Source: CAD feature listing. Evaluate the final solid. Frame: model axes, mm. A direction names the side the tool comes from. Give positions to 0.01 mm unless a question says otherwise; leave off trailing zeros. Order: outer loops, then holes, each group sorted by start corner. A loop starts at its lowest first (then second) coordinate and runs counter-clockwise, first axis right, second up. Notation, with made-up numbers: (16.25, -18) - (73.25, -18) arc R30 ccw to (73.25, 18) - close; hole circle Ø7 at (-32, 21). An arc over 180 degrees is marked (long way). Write each question's results on one line, items separated by ' | '. Start each with the question number.
Item 1: Line query: line 1 along Z through (x, y) = (-95.5, 4); line 2 along Z through (x, y) = (-545, 9.5); line 3 along X through (y, z) = (5.5, -281.5). Output: solid intervals per line, ascending.
Item 2: Section D-D on y = 7.75. Output: boundary loops of the cut face in (x, z).
Item 3: Contact query for flat-ended pins moving along their axis: pin 1 Ø7.5 at (x, y) = (-285.5, 11) entering from +Z; pin 2 Ø1 at (x, y) = (-388.5, 12.5) entering from +Z. Output: stop coordinate, or through.
Item 4: Section C-C on x = -481.5. Output: boundary loops of the cut face in (y, z).
Item 5: Section A-A on x = -389.5. Output: boundary loops of the cut face in (y, z), and give its area (3 significant figures).
Item 6: Set-up query: faces 1 (the cylindrical face through (-172.518, 7.465, -167.871)), 2 (the flat face through (-540, 7, -25)), 3 (the flat face through (-322, 8, -475)). Return all of +Z, -Z, +X, -X, +Y, -Y with unobstructed straight access to the full face (end or side cutting, diameter ignored); none if empty.
Item 7: Mould query, pull axis X, two halves, no side actions, for faces 4 (the flat face through (-167, 0, -170)), 5 (the flat face through (-36.438, 8, -331)), 6 (the flat face through (-609, 7, -257)). Classes: released by +X, released by -X, zero draft, split by the parting line, or undercut.
Item 8: Section B-B on z = -294. Output: boundary loops of the cut face in (x, y), and give its area (3 significant figures).
Autodesk Fusion 360 part; units mm, degrees
sketch "Sketch1" plane through (0, 0, 0) normal (0, 1, 0) x (1, 0, 0)
  line L0 (-25, 25) -> (-25, 482)
  line L1 (-25, 482) -> (-609, 482)
  line L2 (-609, 482) -> (-609, 25)
  line L3 (-609, 25) -> (-469, 25)
  line L4 (-444, 175) -> (-190, 175)
  line L5 (-469, 25) -> (-469, 150)
  arc A0 (-444, 175) -> (-469, 150) centre (-444, 150) ccw
  line L6 (-165, 25) -> (-25, 25)
  line L7 (-165, 150) -> (-165, 25)
  arc A1 (-165, 150) -> (-190, 175) centre (-190, 150) ccw
  point P0 (-469, 175)
  point P1 (-165, 175)
  dimension "d1" = 457
  dimension "d2" = 584
  dimension "d3" = 457
  dimension "d5" = 304
  dimension "d7" = 25
  dimension "d8" = 25
extrude "Extrude1" add sketch "Sketch1" along normal blind 15
sketch "Sketch2" plane through (0, 15, 0) normal (0, 1, 0) x (-1, 0, 0)
  line L0 (165, -25) -> (25, -25)
  line L1 (25, -25) -> (25, -482)
  line L2 (25, -482) -> (609, -482)
  line L3 (609, -482) -> (609, -25)
  line L4 (609, -25) -> (469, -25)
  line L5 (469, -25) -> (469, -150)
  arc A0 (444, -175) -> (469, -150) centre (444, -150) ccw
  line L6 (444, -175) -> (190, -175)
  arc A1 (165, -150) -> (190, -175) centre (190, -150) ccw
  line L7 (165, -150) -> (165, -25)
  line L8 (600, -475) -> (36.4384, -475)
  line L9 (36.4384, -475) -> (36.4384, -182.5461)
  line L10 (36.4384, -182.5461) -> (600, -182.5461)
  line L11 (600, -182.5461) -> (600, -475)
  dimension "d11" = 563.5616
extrude "Extrude2" cut sketch "Sketch2" against normal blind 10 contours L8 L9 L10 L11
shell "Shell1" thickness 5 removed faces 1 at (-412.1461, 5, -377.5154)
extrude "Extrude3" cut 1 faces at (-412.1461, 5, -377.5154) along direction (0, -1, 0) blind 5
sketch "Sketch3" plane through (0, 15, 0) normal (0, 1, 0) x (-1, 0, 0)
  line L0 (36.4384, -475) -> (36.4384, -182.5461)
  line L1 (36.4384, -182.5461) -> (600, -182.5461)
  line L2 (600, -182.5461) -> (600, -475)
  line L3 (600, -475) -> (36.4384, -475)
  line L4 (165, -25) -> (25, -25)
  line L5 (25, -25) -> (25, -482)
  line L6 (25, -482) -> (609, -482)
  line L7 (609, -482) -> (609, -25)
  line L8 (609, -25) -> (469, -25)
  line L9 (469, -25) -> (469, -150)
  arc A0 (444, -175) -> (469, -150) centre (444, -150) ccw
  line L10 (444, -175) -> (190, -175)
  arc A1 (165, -150) -> (190, -175) centre (190, -150) ccw
  line L11 (165, -150) -> (165, -25)
  circle A2 centre (544.2965, -92.6642) radius 50
  curve A3
  dimension "d17" = 100
  dimension "d18" = 100
extrude "Extrude4" cut sketch "Sketch3" against normal blind 20 contours A2
sketch "Sketch4" plane through (0, 15, 0) normal (0, 1, 0) x (-1, 0, 0)
  circle A0 centre (544.2965, -92.6642) radius 50
  line L0 (36.4384, -475) -> (36.4384, -182.5461)
  line L1 (36.4384, -182.5461) -> (600, -182.5461)
  line L2 (600, -182.5461) -> (600, -475)
  line L3 (600, -475) -> (36.4384, -475)
  line L4 (165, -25) -> (25, -25)
  line L5 (25, -25) -> (25, -482)
  line L6 (25, -482) -> (609, -482)
  line L7 (609, -482) -> (609, -25)
  line L8 (609, -25) -> (469, -25)
  line L9 (469, -25) -> (469, -150)
  arc A1 (444, -175) -> (469, -150) centre (444, -150) ccw
  line L10 (444, -175) -> (190, -175)
  arc A2 (165, -150) -> (190, -175) centre (190, -150) ccw
  line L11 (165, -150) -> (165, -25)
  circle A3 centre (92.6724, -96.5653) radius 50
  dimension "d23" = 100
extrude "Extrude5" cut sketch "Sketch4" against normal blind 20 contours A3
fillet "Fillet1" radius 5 1 edges at (-46.056, 0, -114.6461)
fillet "Fillet2" radius 5 1 edges at (-46.056, 15, -78.4846)
fillet "Fillet3" radius 5 1 edges at (-497.6801, 0, -110.745)
fillet "Fillet4" radius 5 1 edges at (-497.6801, 15, -74.5834)
fillet "Fillet5" radius 5 5 edges at (-469, 15, -87.5) (-461.6777, 15, -167.6777) (-317, 15, -175) (-172.3223, 15, -167.6777) (-165, 15, -87.5)
fillet "Fillet6" radius 5 5 edges at (-469, 0, -87.5) (-461.6777, 0, -167.6777) (-317, 0, -175) (-172.3223, 0, -167.6777) (-165, 0, -87.5)
Evaluation:
1) line 1: z = -482 to -475, -182.55 to -146.59, -46.54 to -25 | line 2: z = -482 to -475, -182.55 to -142.66, -42.67 to -25 | line 3: x = -609 to -600, -36.44 to -25
2) outline: (-609, -482) - (-25, -482) - (-25, -25) - (-165, -25) - (-165, -150) arc R25 cw to (-190, -175) - (-444, -175) arc R25 cw to (-469, -150) - (-469, -25) - (-609, -25) - close; hole (-600, -475) - (-36.44, -475) - (-36.44, -182.55) - (-600, -182.55) - close; hole circle Ø100 at (-544.3, -92.66); hole circle Ø100 at (-92.67, -96.57)
3) pin 1: stops at z = -175 | pin 2: stops at z = -175.42
4) outline: (0, -482) - (15, -482) - (15, -475) - (0, -475) - close; (0, -182.55) - (15, -182.55) - (15, -25) - (0, -25) - close
5) outline: (0, -482) - (15, -482) - (15, -475) - (0, -475) - close; (0, -182.55) - (15, -182.55) - (15, -180) arc R5 ccw to (10, -175) - (5, -175) arc R5 ccw to (0, -180) - close | area: 207 mm^2
6) face 1: +Z, +Y, -Y | face 2: +Z, +X, -X, +Y, -Y | face 3: +Y, -Y
7) face 4: zero draft | face 5: undercut | face 6: released by -X
8) outline: (-609, 0) - (-600, 0) - (-600, 15) - (-609, 15) - close; (-36.44, 0) - (-25, 0) - (-25, 15) - (-36.44, 15) - close | area: 307 mm^2
